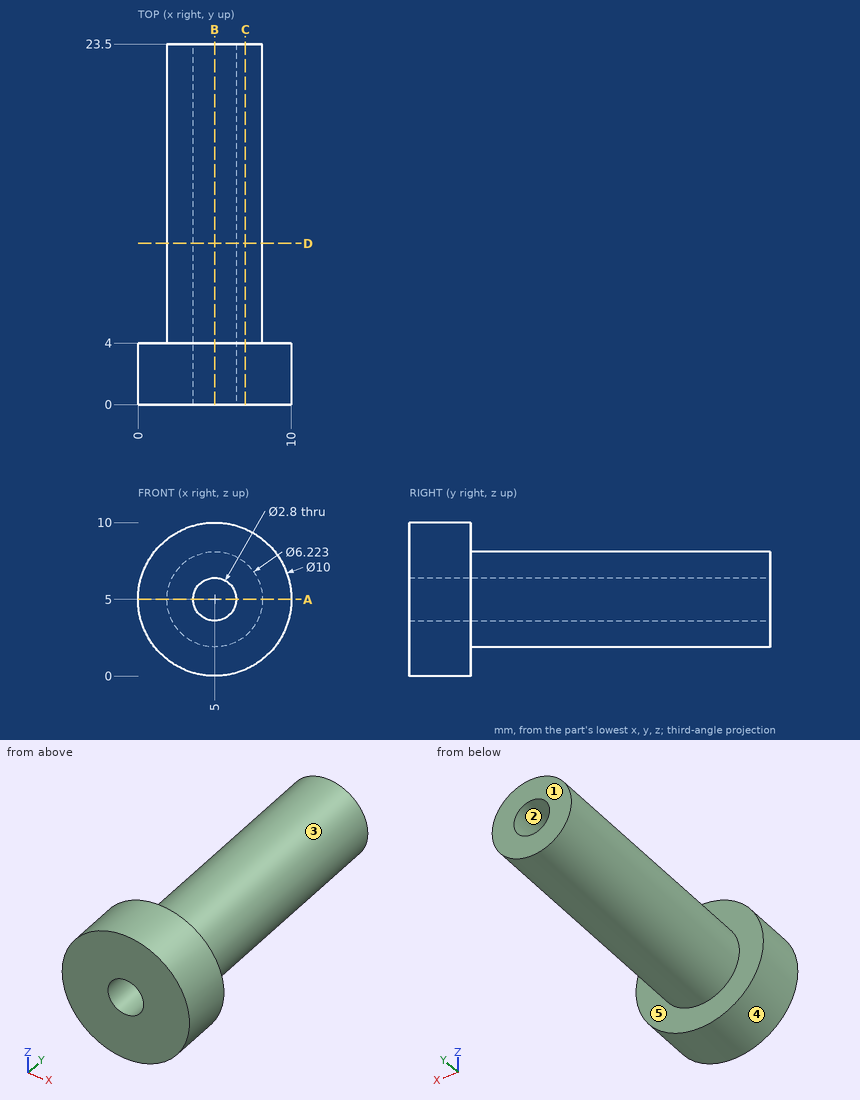
The drawing under review shows one solid part. Ordinate dimensions are in mm from its lowest x, y, z. A direction names the side the tool comes from. Give positions to 0.01 mm unless a question says otherwise; leave off trailing zeros. Write each loop counter-clockwise with the first axis right and the second up, starting at its lowest first coordinate (ties: lowest second). Pieces come first, ordered by that corner, then holes. Notation, with made-up numbers: (-9, 73) -> (13, 73) arc R36 cw to (13, 107) -> close; hole circle Ø1 at (-1, -17). An arc over 180 degrees is marked (long way). Put each result on its own line as item: value.
(1) For pin 1 Ø5 at (y, z) = (7, 3.5) entering from +X; pin 2 Ø2 at (y, z) = (15, 7) entering from +X; pin 3 Ø5 at (x, y) = (8.5, 21) entering from -Z, all flat-tipped, find the tip position at first contact; note any pin that passes through.
Results are:
pin 1: x = 8.11
pin 2: x = 7.95
pin 3: z = 2.05
(2) We need section A-A, the plane z = 5. Give the boundary of the cut face in (x, y), and give its area (3 significant figures).
Results are:
outline: (0, 0) -> (3.6, 0) -> (3.6, 23.5) -> (1.89, 23.5) -> (1.89, 4) -> (0, 4) -> close; (6.4, 0) -> (10, 0) -> (10, 4) -> (8.11, 4) -> (8.11, 23.5) -> (6.4, 23.5) -> close
area: 95.5 mm²
(3) We need section B-B, the plane x = 5. Give the boundary of the cut face in (y, z).
Results are:
outline: (0, 0) -> (4, 0) -> (4, 1.89) -> (23.5, 1.89) -> (23.5, 3.6) -> (0, 3.6) -> close; (0, 6.4) -> (23.5, 6.4) -> (23.5, 8.11) -> (4, 8.11) -> (4, 10) -> (0, 10) -> close
(4) Tool access review of the marked faces 4 and 5: name each direction out of +Z, -Z, +X, -X, +Y, -Y from which nothing blocks a thin tool from reaching the whole face with its end or side.
Results are:
face 4: +Y, -Y
face 5: +Y
(5) We need section D-D, the plane y = 10.5. Give the boundary of the cut face in (x, z).
Results are:
outline: circle Ø6.22 at (5, 5); hole circle Ø2.8 at (5, 5)
(6) We need section C-C, the plane x = 7. Give the boundary of the cut face in (y, z), and give its area (3 significant figures).
Results are:
outline: (0, 0.42) -> (4, 0.42) -> (4, 2.62) -> (23.5, 2.62) -> (23.5, 7.38) -> (4, 7.38) -> (4, 9.58) -> (0, 9.58) -> close
area: 130 mm²
(7) To check wall thickness, follow probe 1 along Z at (x, y) = (5, 13.5); probe 2 along Y at (x, z) = (6, 8.75). State the ranges of each line that lie inside material, in increasing order. Write a range as from..to.
Results are:
probe 1: 1.89..3.6, 6.4..8.11
probe 2: 0..4
(8) The part is to be moulded in two halves that separate along X. For the marked faces 1, 2 and 3, say which applies: pulls with the +X half, pulls with the -X half, needs draft (parallel to the pull), parting line crosses it, or undercut.
Results are:
face 1: needs draft
face 2: undercut
face 3: parting line crosses it
